Check sheet for the drawn part. Datum: minimum x, y, z corner. Units: mm. A direction names the side the tool comes from. Round coordinates to 2 decimals unless told otherwise and drop trailing zeros. Write each loop counter-clockwise with the first axis right and the second up, starting at its lowest first coordinate (ties: lowest second). Pieces come first, ordered by that corner, then holes. Notation, with made-up numbers: (-24, 10.5) - (-16, 10.5) arc R14 ccw to (-16, 18.5) - close; hole circle Ø11 at (-33, 5). An arc over 180 degrees is marked (long way). Answer as a JSON object with one key per item and string values. Group by question number.
Item 1: Sectioned sample at C-C on z = 23. Record the boundary of the cut face in (x, y), plus the area to 3 significant figures.
Item 2: Thickness scan on line 1 (Z direction, x = 4.05, y = 14); line 2 (Z direction, x = 23.5, y = 15.75); line 3 (Z direction, x = 14.5, y = 21.25). Record the ranges inside material, lowest first.
Item 3: Gauge pin test, flat ends, axial feed: P1, Ø4, axis at x = 10.5, y = 3.5, coming from the -Z side; P2, Ø4, axis at y = 13, z = 13.5, coming from the -X side; P3, Ø3, axis at x = 16, y = 19, coming from the -Z side; P4, Ø5.5, axis at y = 14, z = 9.92, coming from the +X side. Record the tip position at first contact, or that the pin passes through.
Item 4: Sectioned sample at B-B on z = 11.5. Record the boundary of the cut face in (x, y), plus the area to 3 significant figures.
Item 5: Sectioned sample at A-A on y = 14. Record the boundary of the cut face in (x, z).
Item 6: Release check for a two-part mould opening along Y. For the marked faces 1, 2 and 3 record: pulls with the +Y half, pulls with the -Y half, needs draft (parallel to the pull), parting line crosses it, or undercut.
Item 7: Set-up check for the marked faces 4 and 5: record each of +Z, -Z, +X, -X, +Y, -Y from which the full face is reachable in a straight line by a thin tool's end or side.
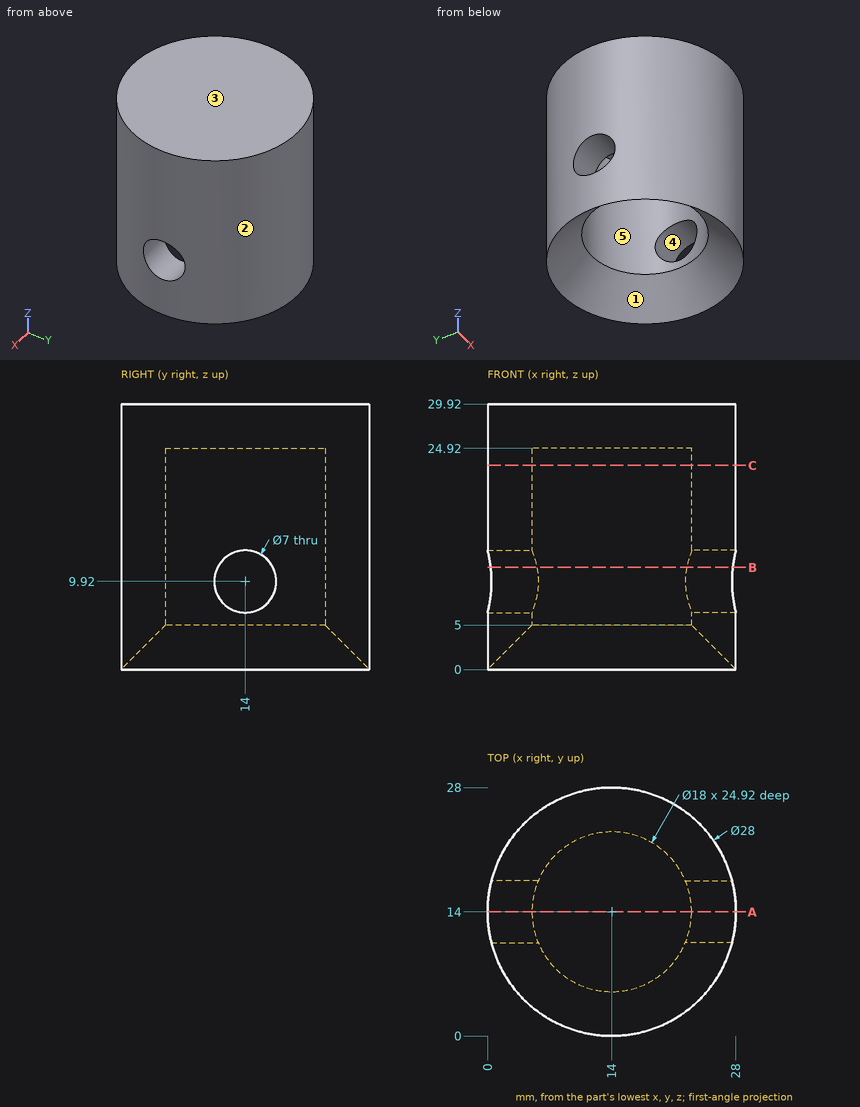
Completed:
{
 "1": {"outline": "circle Ø28 at (14, 14); hole circle Ø18 at (14, 14)", "area": "361 mm²"},
 "2": {"line 1": "4.05 to 6.42, 13.42 to 29.92", "line 2": "4.34 to 6.89, 12.95 to 29.92", "line 3": "24.92 to 29.92"},
 "3": {"P1": "z = 0.93", "P2": "x = 0", "P3": "z = 24.92", "P4": "through"},
 "4": {"outline": "(0.35, 10.88) arc R14 ccw to (27.65, 10.88) - (22.44, 10.88) arc R9 cw to (5.56, 10.88) - close; (0.35, 17.12) - (5.56, 17.12) arc R9 cw to (22.44, 17.12) - (27.65, 17.12) arc R14 ccw to start", "area": "298 mm²"},
 "5": {"outline": "(0, 0) - (5, 5) - (5, 6.42) - (0, 6.42) - close; (0, 13.42) - (5, 13.42) - (5, 24.92) - (23, 24.92) - (23, 13.42) - (28, 13.42) - (28, 29.92) - (0, 29.92) - close; (23, 5) - (28, 0) - (28, 6.42) - (23, 6.42) - close"},
 "6": {"face 1": "undercut", "face 2": "parting line crosses it", "face 3": "needs draft"},
 "7": {"face 4": "+X, -X", "face 5": "-Z"}
}
